from build123d import *

# Parameters (mm, degrees)
F0_W     = 15
F0_H     = 15
F0_W_2   = 10.51
F0_H_2   = 10.51
F1_DEPTH = 25
F2_W     = 15
F2_H     = 15
F3_DEPTH = 25
F4_W     = 15
F4_H     = 15
F5_DEPTH = 70
F6_R     = 5


with BuildPart() as f1:
    # F0 (on Top) → F1 (new body)
    with BuildSketch(Plane.XY):
        Rectangle(F0_W, F0_H)
        Rectangle(F0_W_2, F0_H_2, mode=Mode.SUBTRACT)
    extrude(amount=F1_DEPTH)

    # F2 (on face) → F3 (join)
    with BuildSketch(Plane.XY.offset(25)):
        Rectangle(F2_W, F2_H)
    extrude(amount=F3_DEPTH)

    # F4 (on face) → F5 (join)
    with BuildSketch(Plane(origin=(-7.5, 0, 0), x_dir=(0, -1, 0), z_dir=(-1, 0, 0))):
        with Locations((0, 42.5)):
            Rectangle(F4_W, F4_H)
    extrude(amount=F5_DEPTH)

    # F6
    f6_edges = [f1.edges().sort_by_distance(p)[0] for p in [
        (-35, 7.5, 50),
        (7.5, 0, 50),
        (-35, -7.5, 50),
        (7.5, -7.5, 25),
        (7.5, 7.5, 25),
        (-77.5, 0, 50),
        (-77.5, 7.5, 42.5),
        (-77.5, 0, 35),
        (-77.5, -7.5, 42.5),
        (-42.5, 7.5, 35),
        (-7.5, 7.5, 17.5),
        (-7.5, -7.5, 17.5),
        (-42.5, -7.5, 35),
        (-7.5, 0, 35),
    ]]
    fillet(f6_edges, radius=F6_R)


solid = f1.part
Check sheet for the modelled part. Datum: model origin and axes. Units: mm. A direction names the side the tool comes from. Round coordinates to 2 decimals unless told otherwise and drop trailing zeros. Loops run counter-clockwise (first coordinate to the right, second up) from the corner with the lowest first, then second, coordinate; pieces in that order, holes last. Notation, with made-up numbers: (-25.75, 49.25) - (-10.75, 49.25) arc R17 ccw to (-10.75, 78.25) - close; hole circle Ø1 at (-30.5, 25). An arc over 180 degrees is marked (long way). Answer as CSV lines item,"result". Start each with the question number.
Item 1: Section check B-B (z = 27.5). Record the boundary of the cut face in (x, y), and give its area (3 significant figures).
Item 2: Section check D-D (y = 1). Record the boundary of the cut face in (x, z) (3 decimals), and give its area (3 significant figures).
Item 3: Scan lines: line 1 (Z direction, x = -3.5, y = -0.25); line 2 (X direction, y = -4.25, z = 20.5) (3 decimals); line 3 (X direction, y = 4.5, z = 10.5) (3 decimals). Record each from-to range of solid material in increasing order. Write a range as [from, to].
Item 4: Section check C-C (x = -19.5). Record the boundary of the cut face in (y, z).
Item 5: Release check for a two-part mould opening along Y. For faces 1 (the flat face through (7.5, 0, 22)), 2 (the cylindrical face through (-76, -6.07, 42.54)), 3 (the flat face through (0, 0, 25)) record: +Y half, -Y half, draft (parallel to the pull), parting line (faces both ways), or undercut.
Item 6: Set-up check for faces 4 (the flat face through (0, -5.255, 12)), 5 (the cylindrical face through (-6, 6.07, 14.79)), 6 (the flat face through (-42, 0, 35)), 7 (the cylindrical face through (-42.92, -6.07, 36.5)): record each of +Z, -Z, +X, -X, +Y, -Y from which the full face is reachable in a straight line by a thin tool's end or side.
Item 7: Depth check by flat-ended pin: P1, Ø1.5, axis at x = -57.5, y = -0.5, coming from the -Z side; P2, Ø3, axis at x = 2.5, y = -2, coming from the -Z side; P3, Ø1, axis at y = -1.5, z = 23, coming from the -X side. Enter the tip coordinate at first touch or a pass-through.
Item 8: Section check A-A (z = 5). Record the boundary of the cut face in (x, y) (3 decimals), and give its area (3 significant figures).
Report:
1,outline,"(-7.5, -2.5) arc R5 ccw to (-2.5, -7.5) - (2.5, -7.5) arc R5 ccw to (7.5, -2.5) - (7.5, 2.5) arc R5 ccw to (2.5, 7.5) - (-2.5, 7.5) arc R5 ccw to (-7.5, 2.5) - close"
1,area,"204 mm2"
2,outline,"(-77.5, 40) arc R5 ccw to (-72.5, 35) - (-12.5, 35) arc R5 cw to (-7.5, 30) - (-7.5, 0) - (-5.255, 0) - (-5.255, 25) - (5.255, 25) - (5.255, 0) - (7.5, 0) - (7.5, 45) arc R5 ccw to (2.5, 50) - (-72.5, 50) arc R5 ccw to (-77.5, 45) - close"
2,area,"1,530 mm2"
3,line 1,"z = [25, 50]"
3,line 2,"x = [-7.184, -5.255], [5.255, 7.184]"
3,line 3,"x = [-7.083, -5.255], [5.255, 7.083]"
4,outline,"(-7.5, 40) arc R5 ccw to (-2.5, 35) - (2.5, 35) arc R5 ccw to (7.5, 40) - (7.5, 45) arc R5 ccw to (2.5, 50) - (-2.5, 50) arc R5 ccw to (-7.5, 45) - close"
5,face 1,"draft"
5,face 2,"-Y half"
5,face 3,"undercut"
6,face 4,"-Z"
6,face 5,"-Z, -X, +Y"
6,face 6,"-Z, -X, +Y, -Y"
6,face 7,"-Z, -X, -Y"
7,P1,"stops at z = 35"
7,P2,"stops at z = 25"
7,P3,"stops at x = -7.5"
8,outline,"(-7.5, -2.5) arc R5 ccw to (-2.5, -7.5) - (2.5, -7.5) arc R5 ccw to (7.5, -2.5) - (7.5, 2.5) arc R5 ccw to (2.5, 7.5) - (-2.5, 7.5) arc R5 ccw to (-7.5, 2.5) - close; hole (-5.255, -5.255) - (5.255, -5.255) - (5.255, 5.255) - (-5.255, 5.255) - close"
8,area,"93.1 mm2"
